from build123d import *

# Parameters (mm, degrees)
SKETCH1_W           = 31.5
SKETCH1_H           = 9.5
BOSS_EXTRUDE1_DEPTH = 5
BOSS_EXTRUDE2_DEPTH = 7
CUT_EXTRUDE1_START  = 22.75
SKETCH4_R           = 2
CUT_EXTRUDE1_DEPTH  = 7
SKETCH5_R           = 1.3
CUT_EXTRUDE2_DEPTH  = 7
FILLET2_R           = 1


with BuildPart() as part:
    # Sketch1 → Boss-Extrude1 (new body)
    with BuildSketch(Plane.XY):
        Polygon((-15.75, -13.5), (22.75, -13.5), (22.75, 19.5), (-15.75, 19.5), (-19.75, 19.5), (-19.75, -13.5), align=None)
        with Locations((0, 4.75)):
            Rectangle(SKETCH1_W, SKETCH1_H, mode=Mode.SUBTRACT)
    extrude(amount=BOSS_EXTRUDE1_DEPTH)

    # Sketch2 → Boss-Extrude2 (add)
    with BuildSketch(Plane.XY):
        Polygon((-15.75, 19.5), (-35.75, 19.5), (-35.75, -13.5), (-35.75, -22.087493002), (-15.75, -22.087493002), (-15.75, -13.5), (-15.75, 15.5), (15.75, 15.5), (15.75, 0), (15.75, -13.5), (16.597702011, -13.5), (22.75, -13.5), (22.75, 19.5), (15.756062461, 19.5), align=None)
    extrude(amount=BOSS_EXTRUDE2_DEPTH)

    # Sketch4 → Cut-Extrude1 (cut)
    with BuildSketch(Plane(origin=(0, 0, 0), x_dir=(0, 0, -1), z_dir=(1, 0, 0)).offset(CUT_EXTRUDE1_START)):
        with Locations(Location((-3.5, 4.75, 0), (0, 0, 180))):
            Circle(SKETCH4_R)
    extrude(amount=-CUT_EXTRUDE1_DEPTH, mode=Mode.SUBTRACT)

    # Sketch5 → Cut-Extrude2 (cut)
    with BuildSketch(Plane.XY):
        with Locations((-23.75, -13.91)):
            Circle(SKETCH5_R)
        with Locations((-29.25, -6.91)):
            Circle(SKETCH5_R)
    extrude(amount=CUT_EXTRUDE2_DEPTH, mode=Mode.SUBTRACT)

    # Fillet2
    fillet2_edges = [part.edges().sort_by_distance(p)[0] for p in [
        (-15.75, -6.75, 5),
        (0, 15.5, 5),
        (-15.75, 12.5, 5),
        (-15.75, 0, 2.5),
        (-15.75, 9.5, 2.5),
        (-15.75, -3.293746501, 7),
        (0, 0, 5),
        (0, 9.5, 5),
        (-35.75, -1.293746501, 0),
    ]]
    fillet(fillet2_edges, radius=FILLET2_R - 0.0001)  # a hair under: the kernel refuses the full size


solid = part.part
Can you work these out from the model? Positions are in its coordinate system, mm. A direction names the side the tool comes from. Round coordinates to 2 decimals unless told otherwise and drop trailing zeros. Write each loop counter-clockwise with the first axis right and the second up, starting at its lowest first coordinate (ties: lowest second). Pieces come first, ordered by that corner, then holes. Notation, with made-up numbers: M -35.5,-13.75 L -28.5,-13.75 A23 ccw -28.5,4.25 Z; hole C 58.25,22.5 d2. An arc over 180 degrees is marked long. Use a Markdown table: item, result.
Item 1: I want a section at C-C (z = 3). List the corners of the cut face in (x, y) for me.
Found:
| item | result |
|---|---|
| outline | M -35.75,-22.09 L -15.75,-22.09 L -15.75,-13.5 L 22.75,-13.5 L 22.75,2.81 L 15.75,2.81 L 15.75,0 L -14.75,0 A1 cw -15.75,1 L -15.75,8.5 A1 cw -14.75,9.5 L 15.75,9.5 L 15.75,6.69 L 22.75,6.69 L 22.75,19.5 L -35.75,19.5 Z; hole C -29.25,-6.91 d2.6; hole C -23.75,-13.91 d2.6 |
Item 2: I want a section at A-A (x = -29.25). List the corners of the cut face in (y, z) for me, and give its area (3 significant figures).
Found:
| item | result |
|---|---|
| outline | M -22.09,0 L -8.21,0 L -8.21,7 L -22.09,7 Z; M -5.61,0 L 19.5,0 L 19.5,7 L -5.61,7 Z |
| area | 273 mm2 |
Item 3: We'd pull the mould along Y, two halves only. Please class faces 6 (the face through (-6, 19.5, 3)), 7 (the face through (0, 9.5, 2)), 8 (the face through (22.75, 3, 5)), 9 (the face through (3, -13.5, 3)): released by +Y, released by -Y, zero draft, split by the parting line, or undercut.
Found:
| item | result |
|---|---|
| face 6 | released by +Y |
| face 7 | undercut |
| face 8 | zero draft |
| face 9 | released by -Y |
Item 4: I want a section at B-B (y = 4.75). List the corners of the cut face in (x, z) for me.
Found:
| item | result |
|---|---|
| outline | M -35.75,1 A1 ccw -34.75,0 L -15.75,0 L -15.75,6 A1 ccw -16.75,7 L -35.75,7 Z; M 15.75,0 L 22.75,0 L 22.75,1.5 L 15.75,1.5 Z; M 15.75,5.5 L 22.75,5.5 L 22.75,7 L 15.75,7 Z |
Item 5: For pin 1 Ø1.5 at (x, z) = (-11.5, 3) entering from -Y; pin 2 Ø3 at (x, y) = (3, -5) entering from -Z; pin 3 Ø0.8 at (x, z) = (5, 6.5) entering from -Y; pin 4 Ø1.5 at (x, y) = (1.5, 8.5) entering from -Z, each with a flat end and sliding along its axis, tell me the tip position at first contact or that it passes through.
Found:
| item | result |
|---|---|
| pin 1 | stops at y = -13.5 |
| pin 2 | stops at z = 0 |
| pin 3 | stops at y = 15.5 |
| pin 4 | passes through |
Item 6: If I drill on line 1 along Z through (x, y) = (19.5, 4.75); line 2 along Y through (x, z) = (-1, 2); line 3 along Y through (x, z) = (-23.75, 4.25), over which ranges is the centre line in solid material (lowest first)? Write a range as [from, to].
Found:
| item | result |
|---|---|
| line 1 | z = [0, 1.5], [5.5, 7] |
| line 2 | y = [-13.5, 0], [9.5, 19.5] |
| line 3 | y = [-22.09, -15.21], [-12.61, 19.5] |
Item 7: Which directions (+Z, -Z, +X, -X, +Y, -Y) give clear straight access to the entire face, cutting with the end or side of a thin tool? Please do faces 1 (the face through (19.299, 6.702, 3.066)), 2 (the face through (0, 0, 2)), 3 (the face through (15.75, 1, 4)), 4 (the face through (-35.75, -1, 4)), 5 (the face through (0, 13, 5)).
Found:
| item | result |
|---|---|
| face 1 | +X |
| face 2 | +Z, -Z |
| face 3 | +Z |
| face 4 | +Z, -Z, -X, +Y, -Y |
| face 5 | +Z, -Y |
